The listing builds one solid part. Answer for the finished solid, in the listing's coordinates (mm). Coordinates: 2 decimals unless noted, no trailing zeros. Loops run counter-clockwise (first coordinate to the right, second up) from the corner with the lowest first, then second, coordinate; pieces in that order, holes last. Notation, with made-up numbers: (71, 57) - (85, 57) arc R26 cw to (85, 72) - close; hole circle Ø6 at (39.5, 19). An arc over 180 degrees is marked (long way). Return JSON: item names as keys, results as strings. Group by question number.
1. Find the intervals of material crossed by line 1 along Y through (x, z) = (0, 56) (1 decimal); line 2 along X through (y, z) = (-38.5, 20) (3 decimals); line 3 along Y through (x, z) = (3, 43), in increasing order.
2. Section D-D (z = 29) is taken. Write down the section's boundary in (x, y) (3 decimals), and give its area (3 significant figures).
3. Section C-C (y = -38) is taken. Write down the section's boundary in (x, z) (3 decimals).
4. Each of these flat-tipped pins is pushed along its axis until it touches: P1, Ø12.5, axis at y = -30, z = 40.5, coming from the -X side; P2, Ø0.6, axis at x = 2, z = 15, coming from the +Y side; P3, Ø1, axis at x = 1, z = 69, coming from the +Y side. Where does it stop, or does it pass through?
```python
from build123d import *

# Parameters (mm, degrees)
F0_R     = 1.5875
F1_DEPTH = 88.9
F2_W     = 15.672178
F2_H     = 44.45
F3_DEPTH = 12.7


with BuildPart() as f1:
    # F0 (on Top) → F1 (new body)
    with BuildSketch(Plane.XY):
        with BuildLine():
            Line((3.175, -44.45), (3.175, 0))
            ThreePointArc((3.175, 0), (-2.618172, 1.796051), (1.143, -2.962124))
            Line((1.143, -2.962124), (1.143, -44.45))
            Line((1.143, -44.45), (3.175, -44.45))
        make_face()
        Circle(F0_R, mode=Mode.SUBTRACT)
    extrude(amount=F1_DEPTH)

    # F2 (on face) → F3 (cut, symmetric)
    with BuildSketch(Plane(origin=(1.143, 0, 0), x_dir=(0, -1, 0), z_dir=(-1, 0, 0))):
        with Locations((-4.534089, 22.225)):
            Rectangle(F2_W, F2_H)
    extrude(amount=F3_DEPTH, both=True, mode=Mode.SUBTRACT)


solid = f1.part
```
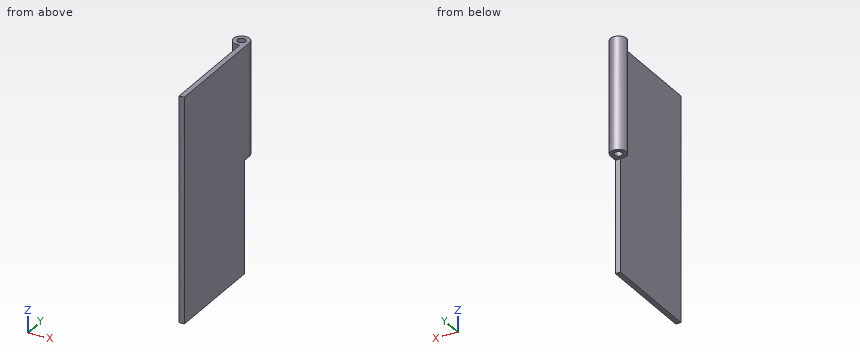
The answers:
{
 "1": {"line 1": "y = -3.2 to -1.6, 1.6 to 3.2", "line 2": "x = 1.143 to 3.175", "line 3": "y = -44.45 to -3.3"},
 "2": {"outline": "(1.143, -44.45) - (3.175, -44.45) - (3.175, -3.302) - (1.143, -3.302) - close", "area": "83.6 mm2"},
 "3": {"outline": "(1.143, 0) - (3.175, 0) - (3.175, 88.9) - (1.143, 88.9) - close"},
 "4": {"P1": "stops at x = 1.14", "P2": "stops at y = -3.3", "P3": "stops at y = 3.14"}
}
